The listing builds one solid part. Answer for the finished solid, in the listing's coordinates (mm). A direction names the side the tool comes from. Give positions to 0.01 mm unless a question says otherwise; leave off trailing zeros. Write each loop counter-clockwise with the first axis right and the second up, starting at its lowest first coordinate (ties: lowest second). Pieces come first, ordered by that corner, then holes. Notation, with made-up numbers: (17, 52.25) -> (65, 52.25) arc R27 cw to (65, 82.25) -> close; hole circle Ø8 at (6.25, 52). An arc over 180 degrees is marked (long way). One line per question, with ' | ' between items.
from build123d import *

# Parameters (mm, degrees)
SKETCH1_W                                            = 35
SKETCH1_H                                            = 140
BOSS_EXTRUDE1_DEPTH                                  = 25
CUT_EXTRUDE1_DEPTH                                   = 144.287298809
CUT_EXTRUDE1_DEPTH_BACK                              = 144.287298809
CBORE_FOR_M3_HEXAGON_SOCKET_HEAD_CAP_SCR_D           = 3.2
CBORE_FOR_M3_HEXAGON_SOCKET_HEAD_CAP_SCR_CBORE_D     = 6
CBORE_FOR_M3_HEXAGON_SOCKET_HEAD_CAP_SCR_CBORE_DEPTH = 18.4
CHAMFER1_SIZE                                        = 2


with BuildPart() as part:
    # Sketch1 → Boss-Extrude1 (new body)
    with BuildSketch(Plane.XY):
        Rectangle(SKETCH1_W, SKETCH1_H)
    extrude(amount=BOSS_EXTRUDE1_DEPTH)

    # Sketch2 → Cut-Extrude1 (cut, two sides: drawn at the far end of the back side and taken through both)
    with BuildSketch(Plane.XZ.offset(70).offset(-CUT_EXTRUDE1_DEPTH_BACK)):
        Polygon((5.5, -90.622577483), (5.5, 0), (5.5, 8), (17.5, 20), (81.579839067, 84.079839067), (247.751789779, 11.714868294), (171.671950713, -162.987548256), align=None)
    extrude(amount=CUT_EXTRUDE1_DEPTH + CUT_EXTRUDE1_DEPTH_BACK, mode=Mode.SUBTRACT)

    # CBORE for M3 Hexagon socket head cap screws1 (through all)
    with Locations(Plane.XY.offset(25)):
        with Locations((-2.5, 65), (-12.5, 0), (-2.5, -65)):
            CounterBoreHole(CBORE_FOR_M3_HEXAGON_SOCKET_HEAD_CAP_SCR_D / 2, CBORE_FOR_M3_HEXAGON_SOCKET_HEAD_CAP_SCR_CBORE_D / 2, CBORE_FOR_M3_HEXAGON_SOCKET_HEAD_CAP_SCR_CBORE_DEPTH)

    # Chamfer1
    chamfer1_edges = [part.edges().sort_by_distance(p)[0] for p in [
        (-17.5, -70, 12.5),
        (-17.5, 70, 12.5),
    ]]
    chamfer(chamfer1_edges, length=CHAMFER1_SIZE)


solid = part.part
Item 1: Find section B-B (y = -65). Write down the section's boundary in (x, z).
Answers below:
outline: (-17.5, 0) -> (-4.1, 0) -> (-4.1, 6.6) -> (-5.5, 6.6) -> (-5.5, 25) -> (-17.5, 25) -> close; (-0.9, 0) -> (5.5, 0) -> (5.5, 8) -> (17.5, 20) -> (17.5, 25) -> (0.5, 25) -> (0.5, 6.6) -> (-0.9, 6.6) -> close
Item 2: Consider line 1 (Y direction, x = -2.5, z = 16.5); line 2 (X direction, y = 65, z = 5.25); line 3 (Y direction, x = -4.5, z = 19). Determine where each line is inside the solid, lowest interval first. Write a range as [from, to].
Answers below:
line 1: [-70, -68], [-62, 62], [68, 70] | line 2: [-17.5, -4.1], [-0.9, 5.5] | line 3: [-70, -67.24], [-62.76, 62.76], [67.24, 70]
Item 3: Find section C-C (z = 15.5). Write down the section's boundary in (x, y).
Answers below:
outline: (-17.5, -68) -> (-15.5, -70) -> (13, -70) -> (13, 70) -> (-15.5, 70) -> (-17.5, 68) -> close; hole circle Ø6 at (-12.5, 0); hole circle Ø6 at (-2.5, -65); hole circle Ø6 at (-2.5, 65)
Item 4: Determine the mould class of faces 4 (the face through (-3, -70, 12)), 5 (the face through (-3.15, -67.93, 15.93)), 6 (the face through (-17.5, -1, 12)) for opening direction Y: pulls with the +Y half, pulls with the -Y half, needs draft (parallel to the pull), parting line crosses it, or undercut.
Answers below:
face 4: pulls with the -Y half | face 5: undercut | face 6: needs draft
Item 5: Flat-ended cylindrical pins translate along their axes: pin 1 (1 mm diameter, centred on x = 6.5, y = -32.5, fed in from -Z); pin 2 (1 mm diameter, centred on y = -29.5, z = 13, fed in from +X); pin 3 (5 mm diameter, centred on x = -2.5, y = -65, fed in from +Z); pin 4 (1.9 mm diameter, centred on x = -12.5, y = 0, fed in from -Z). Find the tip coordinate at first contact, or state that the pin passes through.
Answers below:
pin 1: z = 8.5 | pin 2: x = 11 | pin 3: z = 6.6 | pin 4: through
Item 6: Find section D-D (x = -12.5). Write down the section's boundary in (y, z).
Answers below:
outline: (-70, 0) -> (-1.6, 0) -> (-1.6, 6.6) -> (-3, 6.6) -> (-3, 25) -> (-70, 25) -> close; (1.6, 0) -> (70, 0) -> (70, 25) -> (3, 25) -> (3, 6.6) -> (1.6, 6.6) -> close
Item 7: Find section A-A (x = -2.5). Write down the section's boundary in (y, z).
Answers below:
outline: (-70, 0) -> (-66.6, 0) -> (-66.6, 6.6) -> (-68, 6.6) -> (-68, 25) -> (-70, 25) -> close; (-63.4, 0) -> (63.4, 0) -> (63.4, 6.6) -> (62, 6.6) -> (62, 25) -> (-62, 25) -> (-62, 6.6) -> (-63.4, 6.6) -> close; (66.6, 0) -> (70, 0) -> (70, 25) -> (68, 25) -> (68, 6.6) -> (66.6, 6.6) -> close
Item 8: A tool of negligible diameter and unlimited length cuts with its end or side. For faces 1 (the face through (-11, -1, 6.6)), 2 (the face through (5.5, 1, 4)), 3 (the face through (17.5, -1, 22)), from which of +Z, -Z, +X, -X, +Y, -Y can it reach the whole face along a straight path? Write none if from no direction.
Answers below:
face 1: +Z | face 2: -Z, +X, +Y, -Y | face 3: +Z, -Z, +X, +Y, -Y
